Autodesk Inventor part; units mm, degrees
ref_plane "to_tube_XY" through (3.4671, 0, 0) normal (1, 0, 0) x (0, 0, -1)
ref_plane "to_tube_YZ" through (3.4671, 0, 0) normal (0, 0, -1) x (0, 1, 0)
ref_plane "to_tube_ZX" through (3.4671, 0, 0) normal (0, 1, 0) x (1, 0, 0)
sketch "Sketch_8" plane through (0, 0, 0) normal (0, 0, 1) x (1, 0, 0)
  line L0 (13.5509, 0) -> (0, 0)
  line L1 (0, 0) -> (0, 3.5751)
  line L2 (0, 3.5751) -> (0.508, 4.0831)
  line L3 (0.508, 4.0831) -> (2.9083, 4.0831)
  line L4 (2.9083, 4.0831) -> (3.4671, 3.5242)
  line L5 (3.4671, 3.5242) -> (4.0259, 3.5242)
  line L6 (4.0259, 3.5242) -> (4.0259, 4.3053)
  line L7 (4.0259, 4.3053) -> (4.2799, 4.5593)
  line L8 (4.2799, 4.5593) -> (5.3467, 4.5593)
  line L9 (5.3467, 4.5593) -> (5.3467, 5.3086)
  line L10 (5.3467, 5.3086) -> (5.6007, 5.5626)
  line L11 (5.6007, 5.5626) -> (13.2969, 5.5626)
  line L12 (13.2969, 5.5626) -> (13.5509, 5.3086)
  line L13 (13.5509, 5.3086) -> (13.5509, 0)
  line L14 (13.5509, 0) -> (0, 0)
revolve "Revolution1" add sketch "Sketch_8" angle 360 about axis through (13.5509, 0, 0) along (1, 0, 0)
sketch "Sketch_14" plane through (0, 0, 0) normal (0, 0, 1) x (1, 0, 0)
  line L0 (22.225, 0) -> (13.5509, 0)
  line L1 (13.5509, 0) -> (13.5509, 4.7625)
  line L2 (13.5509, 4.7625) -> (21.5951, 4.7625)
  line L3 (21.5951, 4.7625) -> (22.225, 4.1326)
  line L4 (22.225, 4.1326) -> (22.225, 0)
  line L5 (22.225, 0) -> (13.5509, 0)
revolve "Revolution2" add sketch "Sketch_14" angle 360 about axis through (22.225, 0, 0) along (1, 0, 0)
thread "Thread1"
sketch "Sketch_9" plane through (22.225, 0, 0) normal (1, 0, 0) x (0, 0, -1)
  line L0 (-11.1252, -22.2504) -> (11.1252, -22.2504)
  line L1 (11.1252, -22.2504) -> (11.1252, 22.2504)
  line L2 (11.1252, 22.2504) -> (-11.1252, 22.2504)
  line L3 (-11.1252, 22.2504) -> (-11.1252, -22.2504)
  line L4 (-3.175, -11.1252) -> (3.175, -11.1252)
  line L5 (3.175, -11.1252) -> (3.175, 11.1252)
  line L6 (3.175, 11.1252) -> (-3.175, 11.1252)
  line L7 (-3.175, 11.1252) -> (-3.175, -11.1252)
extrude "Extrusion1" cut sketch "Sketch_9" against normal blind 8.6741
sketch "Sketch_44" plane through (13.5509, 0, 0) normal (1, 0, 0) x (0, 0, -1)
  line L0 (-10.0965, 5.5626) -> (-10.0965, -5.5626)
  line L1 (-10.0965, -5.5626) -> (-4.5339, -5.5626)
  line L2 (-4.5339, -5.5626) -> (-4.5339, 5.5626)
  line L3 (-4.5339, 5.5626) -> (-10.0965, 5.5626)
extrude "Extrusion2" cut sketch "Sketch_44" against normal blind 8.2042
sketch "Sketch5" plane through (0, 0, 0) normal (-1, 0, 0) x (0, 0, 1)
  point P0 (0, 0)
hole "Drilling 1" at (0, 0, 0) direction (1, 0, 0) diameter 3.9675 depth 12.319 tip angle 120
sketch "Sketch6" plane through (5.6007, 3.2228, 4.5339) normal (0, 0, 1) x (1, 0, 0)
  point P0 (3.9243, -3.2228)
hole "Drilling 2" at (9.525, 0, 4.5339) direction (0, 0, -1) diameter 3.9624 depth 4.5339 countersink diameter 4.826 countersink angle 90
sketch "Sketch_24" plane through (0, 0, 0) normal (0, 0, 1) x (1, 0, 0)
  line L0 (4.0259, 0) -> (3.4671, 0)
  line L1 (3.3065, 4.4751) -> (3.9121, 3.8695)
  arc A0 (3.9121, 3.6899) -> (3.9121, 3.8695) centre (3.8223, 3.7797) ccw
  line L2 (3.9121, 3.6899) -> (3.7465, 3.5242)
  line L3 (3.7465, 3.5242) -> (3.4671, 3.5242)
  line L4 (3.4671, 3.5242) -> (3.4671, 3.2702)
  line L5 (3.4671, 3.2702) -> (4.0259, 3.2702)
  line L6 (4.0259, 3.2702) -> (4.0259, 4.0431)
  line L7 (4.0259, 4.0431) -> (3.5097, 4.5593)
  line L8 (3.5097, 4.5593) -> (3.3065, 4.5593)
  line L9 (3.3065, 4.5593) -> (3.3065, 4.4751)
revolve "Revolution3" add sketch "Sketch_24" angle 360 about axis through (4.0259, 0, 0) along (1, 0, 0)
sketch "Sketch_43" plane through (0, 0, 0) normal (0, 0, 1) x (1, 0, 0)
  circle A0 centre (18.2626, 0) radius 2.4066
extrude "Extrusion3" cut sketch "Sketch_43" along normal mid plane 9.525
ref_plane "to_tube_XY" through (3.4671, 0, 0) normal (1, 0, 0) x (0, 0, -1)
ref_plane "to_tube_YZ" through (3.4671, 0, 0) normal (0, 0, -1) x (0, 1, 0)
ref_plane "to_tube_ZX" through (3.4671, 0, 0) normal (0, 1, 0) x (1, 0, 0)
ref_plane "to_nut_XY" through (13.5509, 0, 0) normal (1, 0, 0) x (0, 0, -1)
ref_plane "to_nut_YZ" through (13.5509, 0, 0) normal (0, 0, -1) x (0, 1, 0)
ref_plane "to_nut_ZX" through (13.5509, 0, 0) normal (0, 1, 0) x (1, 0, 0)
ref_plane "lovra1_XY" through (22.225, 0, 0) normal (1, 0, 0) x (0, 0, -1)
ref_plane "lovra1_YZ" through (22.225, 0, 0) normal (0, 0, -1) x (0, 1, 0)
ref_plane "lovra1_ZX" through (22.225, 0, 0) normal (0, 1, 0) x (1, 0, 0)
ref_plane "lovra2_XY" through (22.225, 0, 0) normal (1, 0, 0) x (0, 0, -1)
ref_plane "lovra2_YZ" through (22.225, 0, 0) normal (0, 0, -1) x (0, 1, 0)
ref_plane "lovra2_ZX" through (22.225, 0, 0) normal (0, 1, 0) x (1, 0, 0)
ref_plane "lovra3_XY" through (22.225, 0, 0) normal (1, 0, 0) x (0, 0, -1)
ref_plane "lovra3_YZ" through (22.225, 0, 0) normal (0, 0, -1) x (0, 1, 0)
ref_plane "lovra3_ZX" through (22.225, 0, 0) normal (0, 1, 0) x (1, 0, 0)
ref_plane "to_pin_XY" through (18.2626, 0, 0) normal (0, 0, 1) x (1, 0, 0)
ref_plane "to_pin_YZ" through (18.2626, 0, 0) normal (1, 0, 0) x (0, 1, 0)
ref_plane "to_pin_ZX" through (18.2626, 0, 0) normal (0, 1, 0) x (0, 0, 1)
ref_plane "olen_XY" through (18.2626, 0, 0) normal (1, 0, 0) x (0, 0, -1)
ref_plane "olen_YZ" through (18.2626, 0, 0) normal (0, 0, -1) x (0, 1, 0)
ref_plane "olen_ZX" through (18.2626, 0, 0) normal (0, 1, 0) x (1, 0, 0)
ref_plane "thd1_XY" through (22.225, 0, 4.7625) normal (1, 0, 0) x (0, 0, -1)
ref_plane "thd1_YZ" through (22.225, 0, 4.7625) normal (0, 0, -1) x (0, 1, 0)
ref_plane "thd1_ZX" through (22.225, 0, 4.7625) normal (0, 1, 0) x (1, 0, 0)
ref_plane "p1_XY" through (22.225, 0, 3.175) normal (1, 0, 0) x (0, 0, -1)
ref_plane "p1_YZ" through (22.225, 0, 3.175) normal (0, 0, -1) x (0, 1, 0)
ref_plane "p1_ZX" through (22.225, 0, 3.175) normal (0, 1, 0) x (1, 0, 0)
ref_plane "thd2_XY" through (22.225, 0, -4.7625) normal (1, 0, 0) x (0, 0, -1)
ref_plane "thd2_YZ" through (22.225, 0, -4.7625) normal (0, 0, -1) x (0, 1, 0)
ref_plane "thd2_ZX" through (22.225, 0, -4.7625) normal (0, 1, 0) x (1, 0, 0)
ref_plane "p2_XY" through (22.225, 0, -3.175) normal (1, 0, 0) x (0, 0, -1)
ref_plane "p2_YZ" through (22.225, 0, -3.175) normal (0, 0, -1) x (0, 1, 0)
ref_plane "p2_ZX" through (22.225, 0, -3.175) normal (0, 1, 0) x (1, 0, 0)
ref_plane "port2_XY" through (22.225, 0, 0) normal (1, 0, 0) x (0, 0, -1)
ref_plane "port2_YZ" through (22.225, 0, 0) normal (0, 0, -1) x (0, 1, 0)
ref_plane "port2_ZX" through (22.225, 0, 0) normal (0, 1, 0) x (1, 0, 0)
ref_plane "port_XY" through (9.525, 0, 0) normal (0, 0, 1) x (1, 0, 0)
ref_plane "port_YZ" through (9.525, 0, 0) normal (1, 0, 0) x (0, 1, 0)
ref_plane "port_ZX" through (9.525, 0, 0) normal (0, 1, 0) x (0, 0, 1)
ref_plane "1_XY" through (13.5509, 0, 0) normal (1, 0, 0) x (0, 0, -1)
ref_plane "1_YZ" through (13.5509, 0, 0) normal (0, 0, -1) x (0, 1, 0)
ref_plane "1_ZX" through (13.5509, 0, 0) normal (0, 1, 0) x (1, 0, 0)
ref_plane "lovra21_XY" through (0, 0, 5.2705) normal (1, 0, 0) x (0, 0, -1)
ref_plane "lovra21_YZ" through (0, 0, 5.2705) normal (0, 0, -1) x (0, 1, 0)
ref_plane "lovra21_ZX" through (0, 0, 5.2705) normal (0, 1, 0) x (1, 0, 0)
ref_plane "lovra22_XY" through (0, 0, -5.2705) normal (1, 0, 0) x (0, 0, -1)
ref_plane "lovra22_YZ" through (0, 0, -5.2705) normal (0, 0, -1) x (0, 1, 0)
ref_plane "lovra22_ZX" through (0, 0, -5.2705) normal (0, 1, 0) x (1, 0, 0)
ref_plane "to_screw_XY" through (9.525, 0, 0) normal (0, 1, 0) x (1, 0, 0)
ref_plane "to_screw_YZ" through (9.525, 0, 0) normal (1, 0, 0) x (0, 0, -1)
ref_plane "to_screw_ZX" through (9.525, 0, 0) normal (0, 0, -1) x (0, 1, 0)
ref_plane "to_mounting_bracket_XY" through (13.5509, 0, 0) normal (1, 0, 0) x (0, 0, -1)
ref_plane "to_mounting_bracket_YZ" through (13.5509, 0, 0) normal (0, 0, -1) x (0, 1, 0)
ref_plane "to_mounting_bracket_ZX" through (13.5509, 0, 0) normal (0, 1, 0) x (1, 0, 0)
properties part number "007P0Y000_rear_head"
For this review, take the finished solid that the model builds, in its own axes (mm). A direction names the side the tool comes from. Coordinates: 2 decimals unless noted, no trailing zeros. Write each loop counter-clockwise with the first axis right and the second up, starting at its lowest first coordinate (ties: lowest second). Pieces come first, ordered by that corner, then holes.
(1) Wall thickness on probe 1 along X at (y, z) = (0, 2.5) (3 decimals); probe 2 along Y at (x, z) = (9, 0); probe 3 along Z at (x, y) = (2.75, 0): over which ranges is each line inside the solid? List them lowest first.
(2) For pin 1 Ø6 at (x, z) = (19.5, -1) entering from +Y; pin 2 Ø6.5 at (x, y) = (18.26, 0) entering from +Z (3 decimals); pin 3 Ø4 at (x, z) = (18, -4) entering from -Y, all flat-tipped, find the tip position at first contact; note any pin that passes through.
(3) The part is to be moulded in two halves that separate along Z. For faces 1 (the face through (6.25, -0.09, -1.98)), 2 (the face through (22.225, 0, 0)), 3 (the face through (5.475, -0.197, -5.434)), say which applies: +Z half, -Z half, draft (parallel to the pull), parting line (faces both ways), or undercut.
(4) Tool access review of faces 4 (the face through (16, -2, -3.175)), 5 (the face through (17.629, -4.762, 0.049)), 6 (the face through (5.347, 0, -5)), 7 (the face through (17.629, 4.762, -0.049)): name each direction out of +Z, -Z, +X, -X, +Y, -Y from which nothing blocks a thin tool from reaching the whole face with its end or side.
(5) Add section A-A on x = 4.5. Give the boundary of the cut face in (y, z).
Answer sheet:
1. probe 1: x = 0 to 7.544, 11.506 to 15.856, 20.669 to 22.225
1. probe 2: y = -5.56 to -1.98, 1.98 to 5.56
1. probe 3: z = -4.08 to -1.98, 1.98 to 4.08
2. pin 1: stops at y = 4.76
2. pin 2: stops at z = 3.175
2. pin 3: stops at y = -4.32
3. face 1: undercut
3. face 2: draft
3. face 3: parting line
4. face 4: -Z, +X, +Y, -Y
4. face 5: +X, -Y
4. face 6: -X
4. face 7: +X, +Y
5. outline: circle Ø9.12 at (0, 0); hole circle Ø3.97 at (0, 0)
